For this review, take the finished solid that the model builds, in its own axes (mm). Coordinates: 2 decimals unless noted, no trailing zeros. Loops run counter-clockwise (first coordinate to the right, second up) from the corner with the lowest first, then second, coordinate; pieces in that order, holes last. Notation, with made-up numbers: (86.5, 84.25) -> (101.5, 84.25) arc R31 cw to (101.5, 115.25) -> close; hole circle Ø6 at (55, 4). An arc over 180 degrees is marked (long way). Use a Markdown table: item, result.
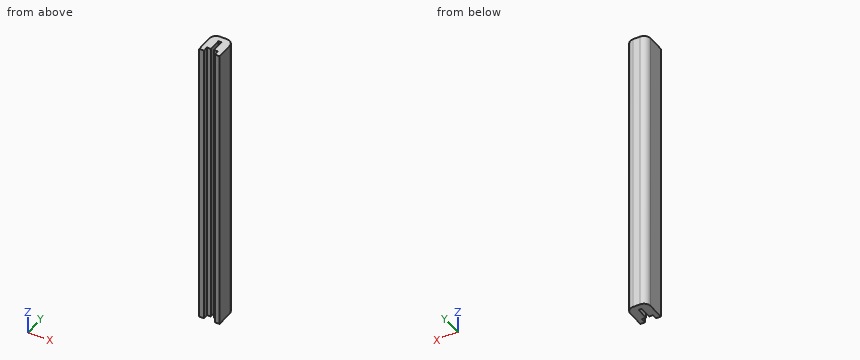
from build123d import *

# Parameters (mm, degrees)
BOSS_EXTRU_1_DEPTH = 430


with BuildPart() as part:
    # Esquisse2 → Boss.-Extru.1 (new body)
    with BuildSketch(Plane.XY):
        with BuildLine():
            Line((-15, 0), (-15, 25))
            ThreePointArc((-15, 25), (-12.071067812, 32.071067812), (-5, 35))
            Line((-5, 35), (5, 35))
            ThreePointArc((5, 35), (12.071067812, 32.071067812), (15, 25))
            Line((15, 25), (15, 0))
            Line((15, 0), (8, 0))
            Line((8, 0), (8, 7.5))
            Line((8, 7.5), (2.25, 7.5))
            Line((2.25, 7.5), (2.25, 26))
            Line((2.25, 26), (-2.25, 26))
            Line((-2.25, 26), (-2.25, 7.5))
            Line((-2.25, 7.5), (-8, 7.5))
            Line((-8, 7.5), (-8, 0))
            Line((-8, 0), (-15, 0))
        make_face()
    extrude(amount=BOSS_EXTRU_1_DEPTH)


solid = part.part
(1) For pin 1 Ø1 at (x, z) = (-2, 144) entering from -Y; pin 2 Ø1.3 at (x, z) = (0, 260) entering from -Y; pin 3 Ø3 at (y, z) = (29.5, 57) entering from -X, all flat-tipped, find the tip position at first contact; note any pin that passes through.
Found:
| item | result |
|---|---|
| pin 1 | stops at y = 7.5 |
| pin 2 | stops at y = 26 |
| pin 3 | stops at x = -14.54 |
(2) Take a section at A-A on y = 20. Write out the cut boundary in (x, z), plus the area to 3 significant figures.
Found:
| item | result |
|---|---|
| outline | (-15, 0) -> (-2.25, 0) -> (-2.25, 430) -> (-15, 430) -> close; (2.25, 0) -> (15, 0) -> (15, 430) -> (2.25, 430) -> close |
| area | 11,000 mm^2 |
(3) For line 1 along X through (y, z) = (23.5, 72); line 2 along X through (y, z) = (6.5, 131); line 3 along Y through (x, z) = (-4, 187.5), list the stretches that pass through material, from the lowest coordinate up.
Found:
| item | result |
|---|---|
| line 1 | x = -15 to -2.25, 2.25 to 15 |
| line 2 | x = -15 to -8, 8 to 15 |
| line 3 | y = 7.5 to 35 |
(4) Take a section at B-B on z = 246.5. Write out the cut boundary in (x, y), plus the area to 3 significant figures.
Found:
| item | result |
|---|---|
| outline | (-15, 0) -> (-8, 0) -> (-8, 7.5) -> (-2.25, 7.5) -> (-2.25, 26) -> (2.25, 26) -> (2.25, 7.5) -> (8, 7.5) -> (8, 0) -> (15, 0) -> (15, 25) arc R10 ccw to (5, 35) -> (-5, 35) arc R10 ccw to (-15, 25) -> close |
| area | 804 mm^2 |
